from build123d import *

# Parameters (mm, degrees)
RESSALTO_EXTRUS_O1_DEPTH = 20
ESBO_O3_R                = 4
CORTE_EXTRUS_O1_DEPTH    = 63.524475359
ESBO_O4_R                = 4
CORTE_EXTRUS_O2_DEPTH    = 84.066238629


with BuildPart() as part:
    # Esboço1 → Ressalto-extrusão1 (new body)
    with BuildSketch(Plane(origin=(0, 0, 0), x_dir=(1, 0, 0), z_dir=(0, 1, 0))):
        Polygon((-70, 36.304347826), (-70, -43.695652174), (10, -43.695652174), (10, -3.695652174), (-30, -3.695652174), (-30, 36.304347826), align=None)
    extrude(amount=RESSALTO_EXTRUS_O1_DEPTH)

    # Esboço3 → Corte-extrusão1 (cut, through all)
    with BuildSketch(Plane(origin=(-30, 0, 0), x_dir=(0, 0, -1), z_dir=(1, 0, 0))):
        with Locations((16.304347826, 10)):
            Circle(ESBO_O3_R)
    extrude(amount=-CORTE_EXTRUS_O1_DEPTH, mode=Mode.SUBTRACT)

    # Esboço4 → Corte-extrusão2 (cut, through all)
    with BuildSketch(Plane(origin=(0, 0, 3.695652174), x_dir=(-1, 0, 0), z_dir=(0, 0, -1))):
        with Locations((10, 10)):
            Circle(ESBO_O4_R)
    extrude(amount=-CORTE_EXTRUS_O2_DEPTH, mode=Mode.SUBTRACT)


solid = part.part
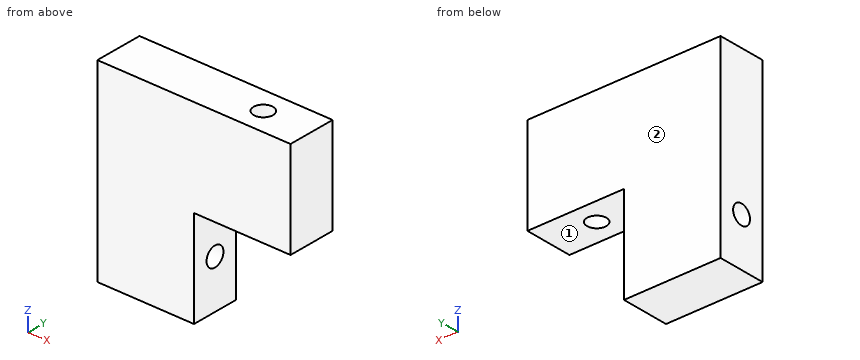
Check sheet for the modelled part. Datum: model origin and axes. Units: mm. Face numbers are marked on the shaded views. A direction names the side the tool comes from. Round coordinates to 2 decimals unless told otherwise and drop trailing zeros. Order: outer loops, then holes, each group sorted by start corner. A loop starts at its lowest first (then second) coordinate and runs counter-clockwise, first axis right, second up. Notation, with made-up numbers: M 36.25,31 L 61.25,31 A26 cw 61.25,51 Z; hole C 29.5,41 d2. An arc over 180 degrees is marked long. One line per item, written item: value. Start each with the question number.
1. Section check C-C on z = 38. Enter the section's corners in (x, y).
2. Section check B-B on y = 10. Enter the section's corners in (x, z), and give its area (3 significant figures).
3. Scan lines: line 1 along Y through (x, z) = (-10, 17.5); line 2 along X through (y, z) = (1, -12); line 3 along Z through (x, y) = (6, 16.75). Record each from-to range of solid material in increasing order.
4. Gauge pin test, flat ends, axial feed: P1, Ø3, axis at x = -22, y = 4.5, coming from the -Z side; P2, Ø6.5, axis at x = -10, y = 10, coming from the -Z side; P3, Ø10, axis at y = 7.5, z = -11, coming from the +X side. Record the tip position at first contact, or that the pin passes through.
5. Section check D-D on x = -37.5. Enter the section's corners in (y, z), and give its area (3 significant figures).
6. Access from +Z, -Z, +X, -X, +Y, -Y to the whole of each face (thin tool, end or side, straight path). Record for the marked faces 1 and 2.
7. Section check A-A on x = -10. Enter the section's corners in (y, z).
Results found:
1. outline: M -70,0 L 10,0 L 10,20 L -70,20 Z; hole C -10,10 d8
2. outline: M -70,-36.3 L -30,-36.3 L -30,-20.3 L -70,-20.3 Z; M -70,-12.3 L -30,-12.3 L -30,3.7 L -14,3.7 L -14,43.7 L -70,43.7 Z; M -6,3.7 L 10,3.7 L 10,43.7 L -6,43.7 Z
2. area: 4,160 mm^2
3. line 1: 0 to 6, 14 to 20
3. line 2: -70 to -30
3. line 3: 3.7 to 43.7
4. P1: z = 3.7
4. P2: through
4. P3: x = -30
5. outline: M 0,-36.3 L 20,-36.3 L 20,43.7 L 0,43.7 Z; hole C 10,-16.3 d8
5. area: 1,550 mm^2
6. face 1: -Z, +X, +Y, -Y
6. face 2: +Z, -Z, +X, -X, +Y
7. outline: M 0,3.7 L 6,3.7 L 6,43.7 L 0,43.7 Z; M 14,3.7 L 20,3.7 L 20,43.7 L 14,43.7 Z
